```python
from build123d import *

# Parameters (mm, degrees)
SKETCH1_R           = 7
BOSS_EXTRUDE1_DEPTH = 3
SKETCH1_3_R         = 4
BOSS_EXTRUDE2_DEPTH = 25
SKETCH3_R           = 0.95
CUT_EXTRUDE1_DEPTH  = 29.19574436
CHAMFER1_SIZE       = 1


with BuildPart() as part:
    # Sketch1 → Boss-Extrude1 (new body)
    with BuildSketch(Plane(origin=(0, 0, 0), x_dir=(1, 0, 0), z_dir=(0, 1, 0))):
        with Locations(Location((0, 0, 0), (0, 0, 270))):
            Circle(SKETCH1_R)
    extrude(amount=-BOSS_EXTRUDE1_DEPTH)

    # Sketch1_3 → Boss-Extrude2 (add)
    with BuildSketch(Plane(origin=(0, 0, 0), x_dir=(1, 0, 0), z_dir=(0, 1, 0))):
        with Locations(Location((0, 0, 0), (0, 0, 270))):
            Circle(SKETCH1_3_R)
    extrude(amount=BOSS_EXTRUDE2_DEPTH)

    # Sketch3 → Cut-Extrude1 (cut, through all)
    with BuildSketch(Plane.ZY.offset(4)):
        with Locations((0, 23)):
            Circle(SKETCH3_R)
    extrude(amount=-CUT_EXTRUDE1_DEPTH, mode=Mode.SUBTRACT)

    # Chamfer1
    chamfer1_edges = [part.edges().sort_by_distance(p)[0] for p in [
        (0, -3, -7),
    ]]
    chamfer(chamfer1_edges, length=CHAMFER1_SIZE)


solid = part.part
```
CAD build for the part. Positions are in the model's coordinates, mm. A direction names the side the tool comes from. Coordinates: 2 decimals unless noted, no trailing zeros. Order: outer loops, then holes, each group sorted by start corner. A loop starts at its lowest first (then second) coordinate and runs counter-clockwise, first axis right, second up. Notation, with made-up numbers: (-38.75, 50) -> (8.25, 50) arc R36 ccw to (8.25, 85) -> close; hole circle Ø8 at (48, -36.75). An arc over 180 degrees is marked (long way). Use one line per item in the form item = value. Start each with the question number.
1) Band-saw the part on C-C on y = 15.75. Give the cut face in (x, z), then the cut area to 3 significant figures.
2) Pull direction Z, two halves, no side cores. Call faces 1 (the cylindrical face through (-3.905, 12.325, -0.867)), 2 (the cylindrical face through (-0.054, 22.073, -0.206)), 3 (the flat face through (0, 25, 0)): +Z half, -Z half, draft (parallel to the pull), parting line (faces both ways), or undercut.
3) Band-saw the part on D-D on y = 23. Give the cut face in (x, z).
4) Drill centre lines: L1, parallel to Y at x = -0.5, z = 0; L2, parallel to Y at x = -1, z = 4.75; L3, parallel to Z at x = -0.5, y = 23. Where is each one in solid material? Low to high. Write a range as [from, to].
5) Band-saw the part on A-A on z = 0. Give the cut face in (x, y).
6) Drop flat-ended pins along their axis: pin 1 (2 mm diameter, centred on y = 3.5, z = -0.5, fed in from +X); pin 2 (6 mm diameter, centred on y = 19.5, z = -4, fed in from -X); pin 3 (3 mm diameter, centred on y = 13, z = -3, fed in from -X). Give the stop position or say it passes through.
7) Tool access for faces 4 (the flat face through (-3, 0, 3)), 5 (the flat face through (0, -3, 0)): list every direction of +Z, -Z, +X, -X, +Y, -Y with a clear straight run to the whole face (end or side of a thin tool).
8) Band-saw the part on B-B on x = 0. Give the cut face in (y, z), then the cut area to 3 significant figures.
Entries:
q1.outline = circle Ø8 at (0, 0)
q1.area = 50.3 mm2
q2.face_1 = parting line
q2.face_2 = undercut
q2.face_3 = draft
q3.outline = (-3.89, -0.95) arc R4 ccw to (3.89, -0.95) -> close; (-3.89, 0.95) -> (3.89, 0.95) arc R4 ccw to start
q4.L1 = [-3, 22.05], [23.95, 25]
q4.L2 = [-3, 0]
q4.L3 = [-3.97, -0.95], [0.95, 3.97]
q5.outline = (-7, -2) -> (-6, -3) -> (6, -3) -> (7, -2) -> (7, 0) -> (4, 0) -> (4, 22.05) -> (-4, 22.05) -> (-4, 0) -> (-7, 0) -> close; (-4, 23.95) -> (4, 23.95) -> (4, 25) -> (-4, 25) -> close
q6.pin_1 = 4
q6.pin_2 = -3.87
q6.pin_3 = -3.71
q7.face_4 = +Y
q7.face_5 = +Z, -Z, +X, -X, -Y
q8.outline = (-3, -6) -> (-2, -7) -> (0, -7) -> (0, -4) -> (25, -4) -> (25, 4) -> (0, 4) -> (0, 7) -> (-2, 7) -> (-3, 6) -> close; hole circle Ø1.9 at (23, 0)
q8.area = 238 mm2
